The figure shows three views and two pictorial views of one solid part (mm, origin at its lowest corner). Answer the questions. A direction names the side the tool comes from. Coordinates: 2 decimals unless noted, no trailing zeros. Write each loop counter-clockwise with the first axis right and the second up, starting at its lowest first coordinate (ties: lowest second). Pieces come first, ordered by that corner, then holes.
Item 1: Straight lines are drawn through the part: probe 1 along Z at (x, y) = (15, 29); probe 2 along Y at (x, z) = (17.1, 29). For each, find the intervals that lie inside material, in ascending order.
Item 2: A tool of negligible diameter and unlimited length cuts with its end or side. For the marked faces 1 and 2, from which of +Z, -Z, +X, -X, +Y, -Y can it reach the whole face along a straight path? Write none if from no direction.
Item 3: Section A-A (x = 14.5) is taken. Give the vertices of the cut face in (y, z), then the cut area to 3 significant figures.
Item 4: Each of these flat-tipped pins is pushed along its axis until it touches: P1, Ø5, axis at y = 52, z = 29, coming from the -X side; P2, Ø5, axis at y = 10.5, z = 6, coming from the +X side; P3, Ø5, axis at x = 2, z = 17, coming from the -Y side; P4, Ø12, axis at x = 7, z = 19.5, coming from the -Y side. Where does it stop, or does it pass through?
Item 5: Section B-B (x = 7) is taken. Give the vertices of the cut face in (y, z), then the cut area to 3 significant figures.
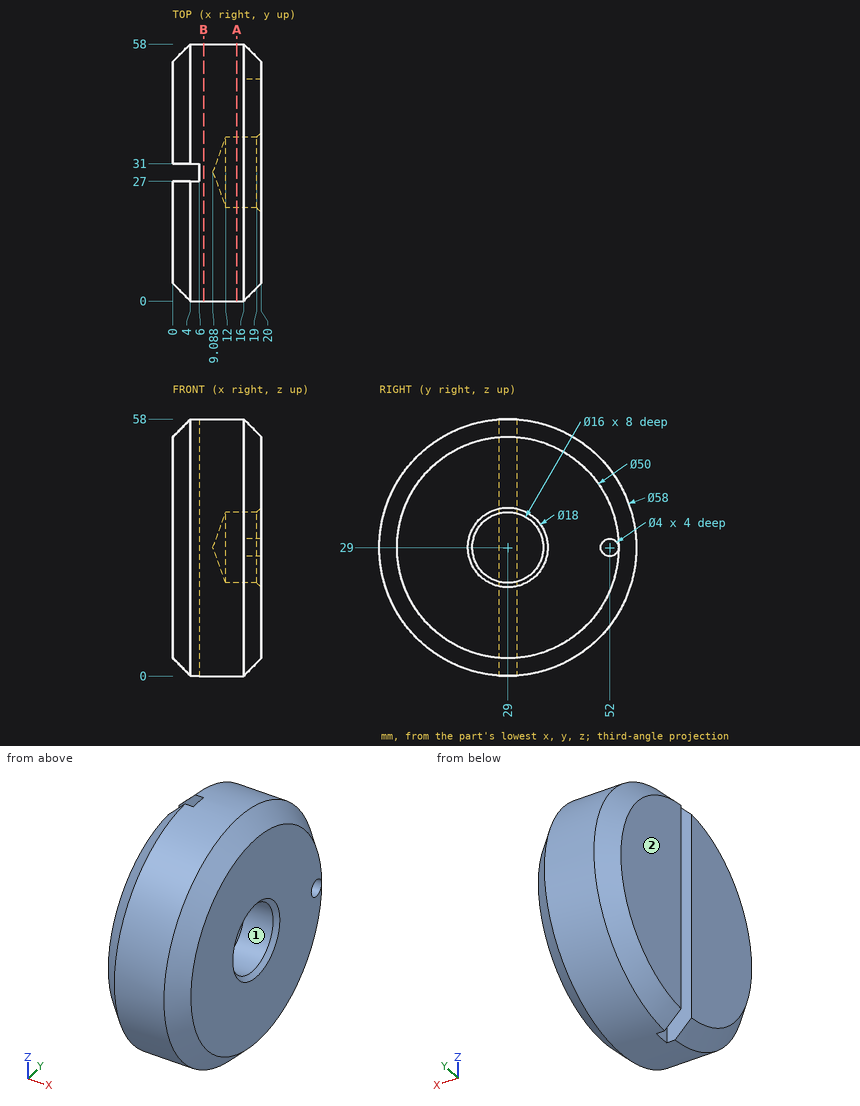
Established:
1. probe 1: z = 0 to 21, 37 to 58
1. probe 2: y = 1.1 to 21, 37 to 50, 54 to 56.9
2. face 1: +X
2. face 2: +Z, -Z, -X, +Y, -Y
3. outline: circle Ø58 at (29, 29); hole circle Ø16 at (29, 29)
3. area: 2,440 mm2
4. P1: stops at x = 0
4. P2: stops at x = 17.98
4. P3: stops at y = 1.97
4. P4: stops at y = 0.21
5. outline: circle Ø58 at (29, 29)
5. area: 2,640 mm2
